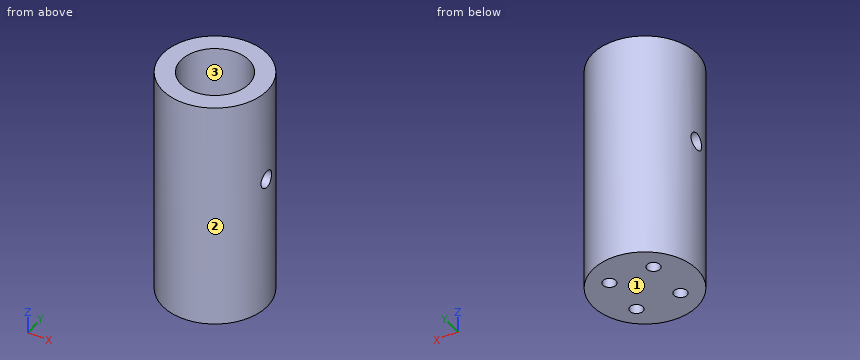
```python
from build123d import *

# Parameters (mm, degrees)
SKETCH_1_R          = 10
EXTRUDE_1_DEPTH     = 44
SKETCH_2_R          = 6.5
CUT_EXTRUDE_1_DEPTH = 27
M4X0_71_D           = 3.3
M3X0_51_D           = 2.5
M3X0_51_DEPTH       = 8.5
M3X0_51_TIP         = 0.751075774


with BuildPart() as part:
    # Эскиз1 → Бобышка-Вытянуть1 (new body)
    with BuildSketch(Plane.XY):
        Circle(SKETCH_1_R)
    extrude(amount=EXTRUDE_1_DEPTH)

    # Эскиз2 → Вырез-Вытянуть1 (cut)
    with BuildSketch(Plane.XY.offset(44)):
        Circle(SKETCH_2_R)
    extrude(amount=-CUT_EXTRUDE_1_DEPTH, mode=Mode.SUBTRACT)

    # Отверстие обработанное метчиком M4x0.71 (through all)
    with Locations(Plane(origin=(-10, 0, 0), x_dir=(0, 0, -1), z_dir=(-1, 0, 0))):
        with Locations((-26, 0)):
            Hole(M4X0_71_D / 2)

    # Отверстие обработанное метчиком M3x0.51
    with Locations(Plane(origin=(0, 0, 0), x_dir=(-1, 0, 0), z_dir=(0, 0, -1))):
        with Locations((-4.242640687, 4.242640687), (4.242640687, 4.242640687), (4.242640687, -4.242640687), (-4.242640687, -4.242640687)):
            Hole(M3X0_51_D / 2, depth=M3X0_51_DEPTH)
            with Locations((0, 0, -(M3X0_51_DEPTH + M3X0_51_TIP / 2))):  # 118° drill point
                Cone(0, M3X0_51_D / 2, M3X0_51_TIP, mode=Mode.SUBTRACT)


solid = part.part
```
Geometry check sheet. Reference: the model listing, model coordinates, mm. Face numbers are marked on the shaded views. Coordinates: 2 decimals unless noted, no trailing zeros. Order: outer loops, then holes, each group sorted by start corner. A loop starts at its lowest first (then second) coordinate and runs counter-clockwise, first axis right, second up. Notation, with made-up numbers: (-31, 33.5) - (27, 33.5) arc R12 cw to (27, 46.5) - close; hole circle Ø3 at (64.5, -14). An arc over 180 degrees is marked (long way). Answer as a JSON object with one key per item and string values. Group by question number.
Item 1: Sectioned sample at B-B, the plane z = 26. Record the cut outline in (x, y).
Item 2: Sectioned sample at D-D, the plane z = 30.5. Record the cut outline in (x, y), and give its area (3 significant figures).
Item 3: Sectioned sample at C-C, the plane x = 0. Record the cut outline in (y, z), and give its area (3 significant figures).
Item 4: Scan lines: probe 1 along X at (y, z) = (0, 23.5); probe 2 along Y at (x, z) = (-4.5, 3); probe 3 along Z at (x, y) = (-1.25, -2). Record each from-to range of solid material in increasing order.
Item 5: Draft check along X on the marked faces 1, 2 and 3. Enter one of: +X half, -X half, draft (parallel to the pull), parting line (faces both ways), or undercut.
Item 6: Sectioned sample at A-A, the plane y = 0. Record the cut outline in (x, z).
Item 7: Depth check by flat-ended pin: pin 1 Ø4 at (x, z) = (-3, 35.5) entering from -Y; pin 2 Ø4 at (x, y) = (3, -1) entering from +Z; pin 3 Ø2 at (y, z) = (6, 30.5) entering from +X; pin 4 Ø2 at (x, y) = (-4.24, 4.24) entering from +Z. Enter the tip coordinate at first touch or a pass-through.
Resolved:
{
 "1": {"outline": "(-9.86, -1.65) arc R10 ccw to (9.86, -1.65) - (6.29, -1.65) arc R6.5 cw to (-6.29, -1.65) - close; (-9.86, 1.65) - (-6.29, 1.65) arc R6.5 cw to (6.29, 1.65) - (9.86, 1.65) arc R10 ccw to start"},
 "2": {"outline": "circle Ø20 at (0, 0); hole circle Ø13 at (0, 0)", "area": "181 mm^2"},
 "3": {"outline": "(-10, 0) - (10, 0) - (10, 44) - (6.5, 44) - (6.5, 17) - (-6.5, 17) - (-6.5, 44) - (-10, 44) - close", "area": "529 mm^2"},
 "4": {"probe 1": "-10 to -6.5, 6.5 to 10", "probe 2": "-8.93 to -5.47, -3.02 to 3.02, 5.47 to 8.93", "probe 3": "0 to 17"},
 "5": {"face 1": "draft", "face 2": "parting line", "face 3": "undercut"},
 "6": {"outline": "(-10, 0) - (10, 0) - (10, 24.35) - (6.5, 24.35) - (6.5, 17) - (-6.5, 17) - (-6.5, 24.35) - (-10, 24.35) - close; (-10, 27.65) - (-6.5, 27.65) - (-6.5, 44) - (-10, 44) - close; (6.5, 27.65) - (10, 27.65) - (10, 44) - (6.5, 44) - close"},
 "7": {"pin 1": "y = -9.95", "pin 2": "z = 17", "pin 3": "x = 8.66", "pin 4": "z = 44"}
}
